Check sheet for the modelled part. Datum: model origin and axes. Units: mm. Face numbers are marked on the shaded views. A direction names the side the tool comes from. Round coordinates to 2 decimals unless told otherwise and drop trailing zeros. Loops run counter-clockwise (first coordinate to the right, second up) from the corner with the lowest first, then second, coordinate; pieces in that order, holes last. Notation, with made-up numbers: (71.25, 17) -> (118.25, 17) arc R27 ccw to (118.25, 40) -> close; hole circle Ø8 at (5.5, 71). An arc over 180 degrees is marked (long way). Use one line per item in the form item = value. Start each with the question number.
(1) Draft check along Z on the marked faces 3, 4, 5 and 6. Enter one of: released by +Z, released by -Z, zero draft, split by the parting line, or undercut.
(2) Sectioned sample at A-A (y = -25.4). Record the cut outline in (x, z) (3 decimals).
(3) Sectioned sample at C-C (y = 28.5). Record the cut outline in (x, z) (3 decimals).
(4) Go/stop test with flat-tipped pins: pin 1 (12 mm diameter, centred on y = -4.5, z = 9, fed in from -X); pin 2 (5 mm diameter, centred on x = 13.5, y = -19, fed in from +Z) (3 decimals); pin 3 (10 mm diameter, centred on x = 11, y = -8.5, fed in from +Z); pin 4 (1.5 mm diameter, centred on x = 12.5, y = 30.5, fed in from -Z). Record where each tip stops, or that it passes through.
(5) Material ranges on probe 1 along Y at (x, z) = (-12.7, 1.5); probe 2 along Y at (x, z) = (-3.5, -1); probe 3 along Z at (x, y) = (-6.5, -29) (3 decimals), recorded low to high. Write a range as [from, to].
(6) Sectioned sample at D-D (z = 9.75). Record the cut outline in (x, y), and give its area (3 significant figures).
(7) Sectioned sample at B-B (x = -11). Record the cut outline in (y, z) (3 decimals), and give its area (3 significant figures).
(8) Set-up check for the marked faces 1 and 2: record each of +Z, -Z, +X, -X, +Y, -Y from which the full face is reachable in a straight line by a thin tool's end or side.
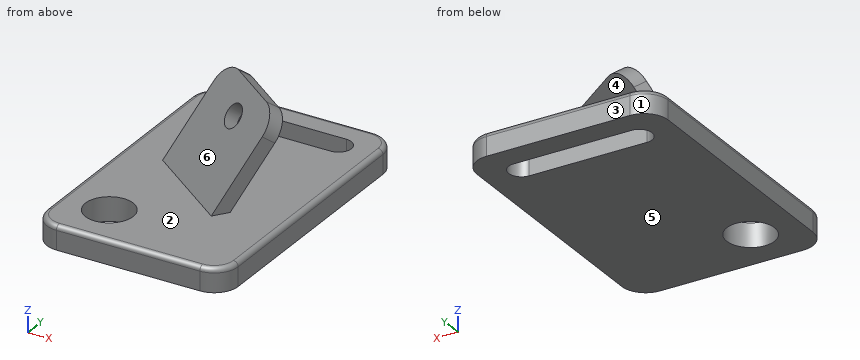
from build123d import *

# Parameters (mm, degrees)
F2_R     = 3.175
F3_DEPTH = 1.905
F0_R     = 6.35
F4_DEPTH = 3.175
F5_R     = 1.27


with BuildPart() as f3:
    # F2 (on face) → F3 (new body, symmetric)
    with BuildSketch(Plane(origin=(-3.023974, -4.077422, 3.55453), x_dir=(0.872864, -0.36782, 0.32065), z_dir=(-0.487963, -0.657953, 0.573576))):
        with BuildLine():
            Line((-3.872431, 23.373911), (-13.813271, 0))
            Line((-13.813271, 0), (13.066727, -11.431966))
            Line((13.066727, -11.431966), (23.007567, 11.941945))
            ThreePointArc((23.007567, 11.941945), (23.05336, 16.801809), (19.649299, 20.270633))
            Line((19.649299, 20.270633), (4.456257, 26.732178))
            ThreePointArc((4.456257, 26.732178), (-0.403607, 26.777972), (-3.872431, 23.373911))
        make_face()
        with Locations((8.822005, 15.904885)):
            Circle(F2_R, mode=Mode.SUBTRACT)
    extrude(amount=F3_DEPTH, both=True)

    # F0 (on Top) → F4 (join, symmetric)
    with BuildSketch(Plane.XY):
        with BuildLine():
            Line((19.05, 38.1), (0, 38.1))
            Line((0, 38.1), (-19.05, 38.1))
            ThreePointArc((-19.05, 38.1), (-23.540128, 36.240128), (-25.4, 31.75))
            Line((-25.4, 31.75), (-25.4, 0))
            Line((-25.4, 0), (-25.4, -31.75))
            ThreePointArc((-25.4, -31.75), (-23.540128, -36.240128), (-19.05, -38.1))
            Line((-19.05, -38.1), (0, -38.1))
            Line((0, -38.1), (19.05, -38.1))
            ThreePointArc((19.05, -38.1), (23.540128, -36.240128), (25.4, -31.75))
            Line((25.4, -31.75), (25.4, 0))
            Line((25.4, 0), (25.4, 31.75))
            ThreePointArc((25.4, 31.75), (23.540128, 36.240128), (19.05, 38.1))
        make_face()
        with Locations((-12.7, -25.4)):
            Circle(F0_R, mode=Mode.SUBTRACT)
        with BuildLine():
            Line((-15.652927, 31.75), (0, 31.75))
            Line((0, 31.75), (15.652927, 31.75))
            ThreePointArc((15.652927, 31.75), (19.05, 28.352927), (15.652927, 24.955855))
            Line((15.652927, 24.955855), (0, 24.955855))
            Line((0, 24.955855), (-15.652927, 24.955855))
            ThreePointArc((-15.652927, 24.955855), (-19.05, 28.352927), (-15.652927, 31.75))
        make_face(mode=Mode.SUBTRACT)
    extrude(amount=F4_DEPTH, both=True)

    # F5
    f5_edges = [f3.edges().sort_by_distance(p)[0] for p in [
        (0, 38.1, 3.175),
        (-23.540128, 36.240128, 3.175),
        (-25.4, 0, 3.175),
        (-23.540128, -36.240128, 3.175),
        (0, -38.1, 3.175),
        (23.540128, -36.240128, 3.175),
        (25.4, 0, 3.175),
        (23.540128, 36.240128, 3.175),
    ]]
    fillet(f5_edges, radius=F5_R)


solid = f3.part
Checks:
q1.face_3 = zero draft
q1.face_4 = undercut
q1.face_5 = released by -Z
q1.face_6 = released by +Z
q2.outline = (-25.4, -3.175) -> (-19.05, -3.175) -> (-19.05, 3.175) -> (-24.13, 3.175) arc R1.27 ccw to (-25.4, 1.905) -> close; (-6.35, -3.175) -> (25.4, -3.175) -> (25.4, 1.905) arc R1.27 ccw to (24.13, 3.175) -> (-6.35, 3.175) -> close
q3.outline = (-25.4, -3.175) -> (-19.047, -3.175) -> (-19.047, 3.175) -> (-24.13, 3.175) arc R1.27 ccw to (-25.4, 1.905) -> close; (19.047, -3.175) -> (25.4, -3.175) -> (25.4, 1.905) arc R1.27 ccw to (24.13, 3.175) -> (19.047, 3.175) -> close
q4.pin_1 = -24.77
q4.pin_2 = 3.175
q4.pin_3 = 20.87
q4.pin_4 = through
q5.probe_1 = [-38.1, -31.75], [-19.05, 24.96], [31.75, 38.1]
q5.probe_2 = [-38.1, 24.96], [31.75, 38.1]
q5.probe_3 = [-3.175, 3.175]
q6.outline = (-12.04, 5.11) -> (11.43, -12.29) -> (14.2, -8.55) -> (-9.26, 8.85) -> close
q6.area = 136 mm2
q7.outline = (-38.1, -3.175) -> (-31.518, -3.175) -> (-31.518, 3.175) -> (-36.83, 3.175) arc R1.27 ccw to (-38.1, 1.905) -> close; (-19.282, -3.175) -> (24.956, -3.175) -> (24.956, 3.175) -> (4.402, 3.175) -> (6.507, 5.59) -> (6.508, 12.233) -> (-1.388, 3.175) -> (-19.282, 3.175) -> close; (31.75, -3.175) -> (38.1, -3.175) -> (38.1, 1.905) arc R1.27 ccw to (36.83, 3.175) -> (31.75, 3.175) -> close
q7.area = 396 mm2
q8.face_1 = +Z, -Z, -X, +Y
q8.face_2 = none
